from build123d import *

# Parameters (mm, degrees)
SKETCH3_R           = 3.5814
CUT_EXTRUDE1_DEPTH  = 5.08
SKETCH4_R           = 6.850820799
BOSS_EXTRUDE1_DEPTH = 20.32
FILLET1_R           = 2.54


# Read off the part's stored shape, not the designer's step: Shell1
with BuildPart() as part:
    # Sketch2 → Revolve1 (revolve)
    with BuildSketch(Plane.XY):
        Polygon((0, 0), (-19.177, 0), (-8.084233452, 177.8), (0, 177.8), align=None)
    revolve(axis=Axis((0, 177.8, 0), (0, -1, 0)))

    # Sketch3 → Cut-Extrude1 (cut)
    with BuildSketch(Plane.XZ):
        Circle(SKETCH3_R)
    extrude(amount=-CUT_EXTRUDE1_DEPTH, mode=Mode.SUBTRACT)

    # Shell1 outline → Shell1 (revolve, cut)
    with BuildSketch(Plane.XY):
        Polygon((6.1214, 7.62), (6.1214, 2.54), (16.473593373, 2.54), (5.697763012, 175.26), (0, 175.26), (0, 7.62), align=None)
    revolve(axis=Axis((0, 0, 0), (0, 1, 0)), mode=Mode.SUBTRACT)

    # Sketch4 → Boss-Extrude1 (add)
    with BuildSketch(Plane(origin=(0, 177.8, 0), x_dir=(1, 0, 0), z_dir=(0, 1, 0))):
        with Locations(Location((0, 0, 0), (0, 0, 180))):
            Circle(SKETCH4_R)
    extrude(amount=BOSS_EXTRUDE1_DEPTH)

    # Fillet1
    # the kernel refuses this fillet: 2.54 mm, written as the material it takes off along each edge
    with BuildSketch(Plane(origin=(0, 198.12, 0), x_dir=(-1, 0, 0), z_dir=(0, 0, -1))) as fillet1_piece_1:
        with BuildLine():
            CenterArc((6.850820799 - FILLET1_R, -FILLET1_R), FILLET1_R, 0, 90)
            Line((6.850820799 - FILLET1_R, 0), (6.850820799 - FILLET1_R, FILLET1_R * 0.02))
            Line((6.850820799 - FILLET1_R, FILLET1_R * 0.02), (6.850820799 + FILLET1_R * 0.02, FILLET1_R * 0.02))
            Line((6.850820799 + FILLET1_R * 0.02, FILLET1_R * 0.02), (6.850820799 + FILLET1_R * 0.02, -FILLET1_R))
            Line((6.850820799 + FILLET1_R * 0.02, -FILLET1_R), (6.850820799, -FILLET1_R))
        make_face()
    revolve(axis=Axis((0, 198.12, 0), (0, 1, 0)), mode=Mode.SUBTRACT)
    with BuildSketch(Plane(origin=(0, 177.8, 0), x_dir=(-1, 0, 0), z_dir=(0, 0, 1))) as fillet1_piece_2:
        with BuildLine():
            CenterArc((5.679920823, 2.254017136), FILLET1_R, 297.450637113, 58.979362887)
            Line((6.850820799, 0), (6.874238798, -0.045080343))
            ThreePointArc((6.874238798, -0.045080343), (7.467527125, -0.0508), (8.084233452, -0.0508))
            Line((8.084233452, -0.0508), (8.134934873, -0.003163212))
            Line((8.134934873, -0.003163212), (8.265693295, 2.092693343))
            Line((8.265693295, 2.092693343), (8.214991874, 2.095856554))
        make_face()
    revolve(axis=Axis((0, 177.8, 0), (0, -1, 0)), mode=Mode.SUBTRACT)


solid = part.part
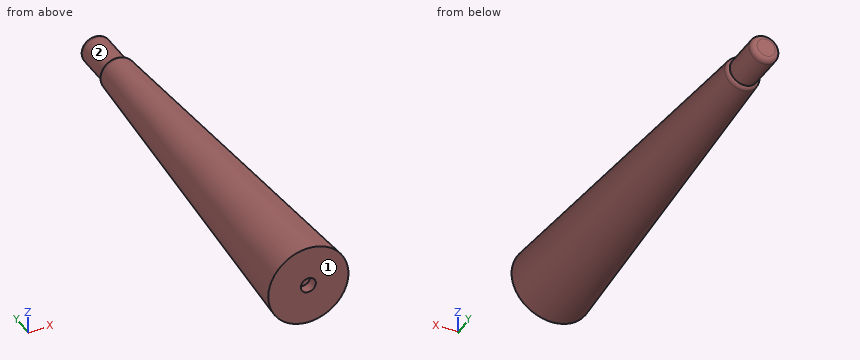
Build history of the part. All positions in model axes, mm. Face numbers are marked on the shaded views. A direction names the side the tool comes from. Coordinates: 2 decimals unless noted, no trailing zeros. Order: outer loops, then holes, each group sorted by start corner. A loop starts at its lowest first (then second) coordinate and runs counter-clockwise, first axis right, second up. Notation, with made-up numbers: (3.5, 1.5) - (28.5, 1.5) arc R14 ccw to (28.5, 20.5) - close; hole circle Ø3 at (66.5, -17.5). An arc over 180 degrees is marked (long way). Write item = value, one per line. Start each with the question number.
1) Wall check: line 1 along Z through (x, y) = (0, 3); line 2 along Y through (x, z) = (1.5, 0.5); line 3 along Z through (x, y) = (0, 1.7). Give the ranges that are in metal, low to high. Write a range as from..to.
2) Flat gauge pins, fed straight in: pin 1 Ø12 at (y, z) = (101, 9) entering from +X; pin 2 Ø1.5 at (x, y) = (5, 100) entering from -Z; pin 3 Ø3 at (y, z) = (29, 7) entering from +X. Where does each tip first touch, or does it go through?
3) Saw through at B-B on z = 0. Write the cut outline in (x, y) (3 decimals), then the cut area to 3 significant figures.
4) Saw through at C-C on y = 114. Write the cut outline in (x, z).
5) 3-axis set-ups, long thin cutter, end or side, ignore diameter. For the marked faces 1 and 2: which of +Z, -Z, +X, -X, +Y, -Y reach the whole face in a straight line?
6) Saw through at D-D on y = 14. Write the cut outline in (x, z), then the cut area to 3 significant figures.
7) Saw through at A-A on x = 0. Write the cut outline in (y, z) (3 decimals), then the cut area to 3 significant figures.
From the geometry:
q1.line_1 = -18.99..-16.44, -6.12..-3.58, 3.58..6.12, 16.44..18.99
q1.line_2 = 5.08..7.62, 175.26..198.12
q1.line_3 = -19.07..-3.58, 3.58..19.07
q2.pin_1 = 12.57
q2.pin_2 = -12.22
q2.pin_3 = 16.48
q3.outline = (-19.177, 0) - (-3.581, 0) - (-3.581, 5.08) - (3.581, 5.08) - (3.581, 0) - (19.177, 0) - (8.215, 175.704) arc R2.54 ccw to (6.851, 177.8) - (6.851, 195.58) arc R2.54 ccw to (4.311, 198.12) - (-4.311, 198.12) arc R2.54 ccw to (-6.851, 195.58) - (-6.851, 177.8) arc R2.54 ccw to (-8.215, 175.704) - close; hole (-16.474, 2.54) - (-6.121, 2.54) - (-6.121, 7.62) - (6.121, 7.62) - (6.121, 2.54) - (16.474, 2.54) - (5.698, 175.26) - (-5.698, 175.26) - close
q3.area = 1,320 mm^2
q4.outline = circle Ø24.13 at (0, 0); hole circle Ø19.04 at (0, 0)
q5.face_1 = +Z, -Z, +X, -X, -Y
q5.face_2 = +Y
q6.outline = circle Ø36.61 at (0, 0); hole circle Ø31.52 at (0, 0)
q6.area = 272 mm^2
q7.outline = (0, -19.177) - (175.704, -8.215) arc R2.54 ccw to (177.8, -6.851) - (195.58, -6.851) arc R2.54 ccw to (198.12, -4.311) - (198.12, 4.311) arc R2.54 ccw to (195.58, 6.851) - (177.8, 6.851) arc R2.54 ccw to (175.704, 8.215) - (0, 19.177) - (0, 3.581) - (5.08, 3.581) - (5.08, -3.581) - (0, -3.581) - close; hole (2.54, -16.474) - (175.26, -5.698) - (175.26, 5.698) - (2.54, 16.474) - (2.54, 6.121) - (7.62, 6.121) - (7.62, -6.121) - (2.54, -6.121) - close
q7.area = 1,320 mm^2
